from build123d import *

# Parameters (mm, degrees)
SKETCH1_W               = 76.2
SKETCH1_H               = 25.4
SKETCH1_W_2             = 70.104
SKETCH1_H_2             = 19.304
BOSS_EXTRUDE1_DEPTH     = 503
SKETCH3_W               = 76.2
SKETCH3_H               = 25.4
SKETCH3_W_2             = 70.104
SKETCH3_H_2             = 19.304
BOSS_EXTRUDE2_DEPTH     = 38.1
CUT_EXTRUDE1_DEPTH      = 13.7
CUT_EXTRUDE1_DEPTH_BACK = 13.7
SKETCH4_W               = 76.2
SKETCH4_H               = 25.4
SKETCH4_W_2             = 70.104
SKETCH4_H_2             = 19.304
BOSS_EXTRUDE3_DEPTH     = 38.1
CUT_EXTRUDE4_DEPTH      = 77.2


with BuildPart() as part:
    # Sketch1 → Boss-Extrude1 (new body)
    with BuildSketch(Plane(origin=(0, 0, 0), x_dir=(1, 0, 0), z_dir=(0, 1, 0))):
        Rectangle(SKETCH1_W, SKETCH1_H)
        Rectangle(SKETCH1_W_2, SKETCH1_H_2, mode=Mode.SUBTRACT)
    extrude(amount=BOSS_EXTRUDE1_DEPTH)

    # Sketch3 → Boss-Extrude2 (add)
    with BuildSketch(Plane.XZ):
        Rectangle(SKETCH3_W, SKETCH3_H)
        Rectangle(SKETCH3_W_2, SKETCH3_H_2, mode=Mode.SUBTRACT)
    extrude(amount=BOSS_EXTRUDE2_DEPTH)

    # Sketch5 → Cut-Extrude1 (cut, two sides)
    with BuildSketch(Plane(origin=(0, 0.04766681, 0), x_dir=(0, -1, 0), z_dir=(0, 0, -1))) as cut_extrude1_sk:
        Polygon((-54.539816916, 54.485087066), (43.408433109, -43.279429016), (134.538834899, 48.02223888), (36.590584874, 145.786754963), align=None)
    extrude(amount=CUT_EXTRUDE1_DEPTH, mode=Mode.SUBTRACT)
    extrude(cut_extrude1_sk.sketch, amount=-CUT_EXTRUDE1_DEPTH_BACK, mode=Mode.SUBTRACT)

    # Sketch4 → Boss-Extrude3 (add)
    with BuildSketch(Plane(origin=(0, 503, 0), x_dir=(1, 0, 0), z_dir=(0, 1, 0))):
        Rectangle(SKETCH4_W, SKETCH4_H)
        Rectangle(SKETCH4_W_2, SKETCH4_H_2, mode=Mode.SUBTRACT)
    extrude(amount=BOSS_EXTRUDE3_DEPTH)

    # Sketch7 → Cut-Extrude4 (cut, through all)
    with BuildSketch(Plane(origin=(38.1, 0, 0), x_dir=(0, 0, -1), z_dir=(1, 0, 0))):
        Polygon((0, 503), (-33.872693161, 487.286257), (-33.967674724, 580.672666523), (15.906824851, 602.541381241), (53.592410045, 527.861836472), align=None)
    extrude(amount=-CUT_EXTRUDE4_DEPTH, mode=Mode.SUBTRACT)


solid = part.part
Source: CAD feature listing. Evaluate the final solid. Frame: model axes, mm. A direction names the side the tool comes from. Coordinates: 2 decimals unless noted, no trailing zeros. Write each loop counter-clockwise with the first axis right and the second up, starting at its lowest first coordinate (ties: lowest second). Pieces come first, ordered by that corner, then holes. Notation, with made-up numbers: M 49,37 L 106,37 A12 ccw 106,58 Z; hole C 4,36.5 d1. An arc over 180 degrees is marked long. Use a Markdown table: item, result.
1) Reachability of faces 5 (the flat face through (-35.052, 268, 0)), 6 (the flat face through (-3.033, 3.039, -10.289)) from +Z, -Z, +X, -X, +Y, -Y: full face, straight path, thin tool, end or side. Return the list, or none.
Conclusion:
| item | result |
|---|---|
| face 5 | +Y, -Y |
| face 6 | +Z, -Z, -X, -Y |
2) Mould query, pull axis X, two halves, no side actions, for faces 1 (the flat face through (-38.1, 270, 0)), 2 (the flat face through (38.1, 232, 0)), 3 (the flat face through (-1, 232, -12.7)), 4 (the flat face through (0, 228, 9.652)). Classes: pulls with the +X half, pulls with the -X half, needs draft (parallel to the pull), parting line crosses it, or undercut.
Conclusion:
| item | result |
|---|---|
| face 1 | pulls with the -X half |
| face 2 | pulls with the +X half |
| face 3 | needs draft |
| face 4 | undercut |
3) Section D-D, the plane x = -25.5. Output: boundary loops of the cut face in (y, z).
Conclusion:
| item | result |
|---|---|
| outline | M 25.55,-12.7 L 508.89,-12.7 L 507.48,-9.65 L 25.55,-9.65 Z; M 25.55,9.65 L 498.52,9.65 L 497.11,12.7 L 25.55,12.7 Z |
4) Section B-B, the plane x = 0. Output: boundary loops of the cut face in (y, z).
Conclusion:
| item | result |
|---|---|
| outline | M 0,-12.7 L 508.89,-12.7 L 507.48,-9.65 L 0,-9.65 Z; M 0,9.65 L 498.52,9.65 L 497.11,12.7 L 0,12.7 Z |
5) Section C-C, the plane z = -4.25. Output: boundary loops of the cut face in (x, y).
Conclusion:
| item | result |
|---|---|
| outline | M -38.1,38.17 L -35.05,35.12 L -35.05,504.97 L -38.1,504.97 Z; M 35.05,-35.12 L 38.03,-38.1 L 38.1,-38.1 L 38.1,504.97 L 35.05,504.97 Z |
6) Ray query, L1, parallel to Z at x = 27, y = 103; L2, parallel to X at y = 175, z = 2; L3, parallel to X at y = 26.5, z = 3.25. Return the intervals inside material, ascending.
Conclusion:
| item | result |
|---|---|
| L1 | z = -12.7 to -9.65, 9.65 to 12.7 |
| L2 | x = -38.1 to -35.05, 35.05 to 38.1 |
| L3 | x = 35.05 to 38.1 |
7) Section A-A, the plane y = 429.5. Output: boundary loops of the cut face in (x, z).
Conclusion:
| item | result |
|---|---|
| outline | M -38.1,-12.7 L 38.1,-12.7 L 38.1,12.7 L -38.1,12.7 Z; hole M -35.05,-9.65 L 35.05,-9.65 L 35.05,9.65 L -35.05,9.65 Z |
8) First-contact query: pin 1 Ø8 at (x, z) = (11.5, -9) entering from +Y; pin 2 Ø6 at (x, z) = (-11.5, 4.5) entering from +Y. Flat tips, straight axial feed; report the tip coordinate or a pass-through.
Conclusion:
| item | result |
|---|---|
| pin 1 | stops at y = 508.89 |
| pin 2 | passes through |
